Check sheet for the modelled part. Datum: model origin and axes. Units: mm. Give positions to 0.01 mm unless a question says otherwise; leave off trailing zeros. Loops run counter-clockwise (first coordinate to the right, second up) from the corner with the lowest first, then second, coordinate; pieces in that order, holes last. Notation, with made-up numbers: (-39.5, 18.5) - (-5.5, 18.5) arc R19 cw to (-5.5, 30.5) - close; hole circle Ø1 at (27.5, 29). An arc over 180 degrees is marked (long way). Use one line per item in the form item = value.
from build123d import *

# Parameters (mm, degrees)
F0_W     = 152.4
F0_H     = 114.3
F1_DEPTH = 6.35
F3_DEPTH = 6.351
F5_D     = 19.05
F6_R     = 12.7
F7_R     = 12.7


with BuildPart() as f1:
    # F0 (on Front) → F1 (new body)
    with BuildSketch(Plane.XZ):
        Rectangle(F0_W, F0_H)
    extrude(amount=F1_DEPTH)

    # F2 (on face) → F3 (cut, through all)
    with BuildSketch(Plane.XZ.offset(6.35)):
        with BuildLine():
            Line((-12.7, 47.625), (-63.5, 47.625))
            ThreePointArc((-63.5, 47.625), (-66.675, 44.45), (-63.5, 41.275))
            Line((-63.5, 41.275), (-12.7, 41.275))
            ThreePointArc((-12.7, 41.275), (-9.525, 44.45), (-12.7, 47.625))
        make_face()
        with BuildLine():
            Line((-12.7, -41.275), (-63.5, -41.275))
            ThreePointArc((-63.5, -41.275), (-66.675, -44.45), (-63.5, -47.625))
            Line((-63.5, -47.625), (-12.7, -47.625))
            ThreePointArc((-12.7, -47.625), (-9.525, -44.45), (-12.7, -41.275))
        make_face()
        with BuildLine():
            ThreePointArc((-63.5, 34.925), (-66.675, 31.75), (-63.5, 28.575))
            Line((-63.5, 28.575), (-12.7, 28.575))
            ThreePointArc((-12.7, 28.575), (-9.525, 31.75), (-12.7, 34.925))
            Line((-12.7, 34.925), (-63.5, 34.925))
        make_face()
        with BuildLine():
            Line((-12.7, -28.575), (-63.5, -28.575))
            ThreePointArc((-63.5, -28.575), (-66.675, -31.75), (-63.5, -34.925))
            Line((-63.5, -34.925), (-12.7, -34.925))
            ThreePointArc((-12.7, -34.925), (-9.525, -31.75), (-12.7, -28.575))
        make_face()
        with BuildLine():
            Line((-12.7, 22.225), (-63.5, 22.225))
            ThreePointArc((-63.5, 22.225), (-66.675, 19.05), (-63.5, 15.875))
            Line((-63.5, 15.875), (-12.7, 15.875))
            ThreePointArc((-12.7, 15.875), (-9.525, 19.05), (-12.7, 22.225))
        make_face()
        with BuildLine():
            Line((-12.7, -15.875), (-63.5, -15.875))
            ThreePointArc((-63.5, -15.875), (-66.675, -19.05), (-63.5, -22.225))
            Line((-63.5, -22.225), (-12.7, -22.225))
            ThreePointArc((-12.7, -22.225), (-9.525, -19.05), (-12.7, -15.875))
        make_face()
        with BuildLine():
            Line((-12.7, 9.525), (-63.5, 9.525))
            ThreePointArc((-63.5, 9.525), (-66.675, 6.35), (-63.5, 3.175))
            Line((-63.5, 3.175), (-12.7, 3.175))
            ThreePointArc((-12.7, 3.175), (-9.525, 6.35), (-12.7, 9.525))
        make_face()
        with BuildLine():
            ThreePointArc((-63.5, -3.175), (-66.675, -6.35), (-63.5, -9.525))
            Line((-63.5, -9.525), (-12.7, -9.525))
            ThreePointArc((-12.7, -9.525), (-9.525, -6.35), (-12.7, -3.175))
            Line((-12.7, -3.175), (-63.5, -3.175))
        make_face()
    extrude(amount=-F3_DEPTH, mode=Mode.SUBTRACT)

    # F5 (through all)
    with Locations(Plane(origin=(0, 0, 0), x_dir=(1, 0, 0), z_dir=(0, 1, 0))):
        with Locations((38.1, 31.75), (38.1, 0), (38.1, -31.75)):
            Hole(F5_D / 2)

    # F6
    f6_edges = [f1.edges().sort_by_distance(p)[0] for p in [
        (76.2, -3.175, 57.15),
        (76.2, -3.175, -57.15),
    ]]
    fillet(f6_edges, radius=F6_R)

    # F7
    f7_edges = [f1.edges().sort_by_distance(p)[0] for p in [
        (-76.2, -3.175, 57.15),
        (-76.2, -3.175, -57.15),
    ]]
    fillet(f7_edges, radius=F7_R)


solid = f1.part
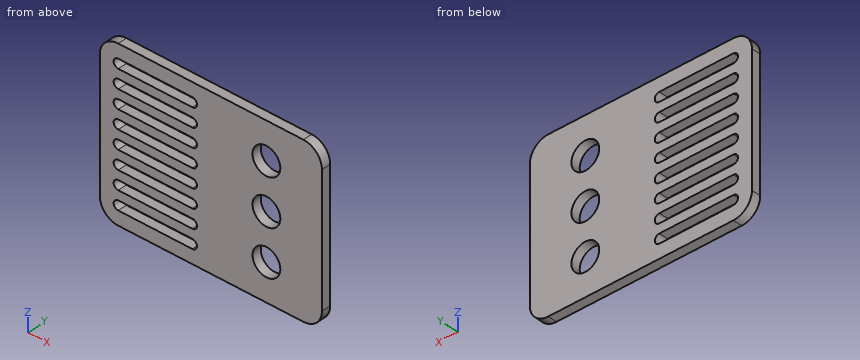
Item 1: Section check A-A on z = 31.75. Record the boundary of the cut face in (x, y) (3 decimals).
Answer block:
outline = (-76.2, -6.35) - (-66.675, -6.35) - (-66.675, 0) - (-76.2, 0) - close; (-9.525, -6.35) - (28.575, -6.35) - (28.575, 0) - (-9.525, 0) - close; (47.625, -6.35) - (76.2, -6.35) - (76.2, 0) - (47.625, 0) - close
Item 2: Thickness scan on L1, parallel to Z at x = 38.1, y = -4.5 (3 decimals); L2, parallel to X at y = -2.75, z = 4; L3, parallel to X at y = -5, z = 20.5. Record the ranges inside material, lowest first.
Answer block:
L1 = -57.15 to -41.275, -22.225 to -9.525, 9.525 to 22.225, 41.275 to 57.15
L2 = -76.2 to -65.63, -10.57 to 29.46, 46.74 to 76.2
L3 = -76.2 to -66.32, -9.88 to 76.2
Item 3: Section check C-C on z = 19.05. Record the boundary of the cut face in (x, y) (3 decimals).
Answer block:
outline = (-76.2, -6.35) - (-66.675, -6.35) - (-66.675, 0) - (-76.2, 0) - close; (-9.525, -6.35) - (76.2, -6.35) - (76.2, 0) - (-9.525, 0) - close
Item 4: Section check B-B on x = 38.1. Record the boundary of the cut face in (y, z) (3 decimals), then the cut area to 3 significant figures.
Answer block:
outline = (-6.35, -57.15) - (0, -57.15) - (0, -41.275) - (-6.35, -41.275) - close; (-6.35, -22.225) - (0, -22.225) - (0, -9.525) - (-6.35, -9.525) - close; (-6.35, 9.525) - (0, 9.525) - (0, 22.225) - (-6.35, 22.225) - close; (-6.35, 41.275) - (0, 41.275) - (0, 57.15) - (-6.35, 57.15) - close
area = 363 mm2
Item 5: Section check D-D on y = -1.75. Give the number of separate pieces and of enclosed holes in the cut face, then the cut area to 3 significant figures.
Answer block:
separate_pieces = 1
enclosed_holes = 11
area = 13,600 mm2
